The model under review builds one solid part; all positions refer to its coordinate system, in mm. Round coordinates to 2 decimals unless told otherwise and drop trailing zeros. Order: outer loops, then holes, each group sorted by start corner. A loop starts at its lowest first (then second) coordinate and runs counter-clockwise, first axis right, second up.
1) Clearance check with flat-ended pins moving along their axes: P1, Ø1, axis at x = 10, z = 38, coming from the +Y side; P2, Ø5, axis at x = 2.5, z = 35, coming from the -Y side; P3, Ø10, axis at x = -1.5, y = 10.5, coming from the +Z side. State where each tip first meets the part, or that it passes through.
2) Mouldability with a two-part tool opening along Y and no side actions: class faces 1 (the face through (0, 0, 0)), 2 (the face through (-29.97, 1.32, 33.28)), 3 (the face through (0, 0, 7)) as pulls with the +Y half, pulls with the -Y half, needs draft (parallel to the pull), parting line crosses it, or undercut.
3) To check wall thickness, follow L1, parallel to Y at x = 0, z = 61; L2, parallel to Z at x = 23, y = 1; L3, parallel to Y at x = 8.5, z = 64. State the ranges of each line that lie inside material, in increasing order.
4) Consider section A-A (x = 0). Give the boundary of the cut face in (y, z).
5) Consider section C-C (z = 58.5). Give the boundary of the cut face in (x, y).
from build123d import *

# Parameters (mm, degrees)
F0_R     = 30
F0_R_2   = 25
F1_DEPTH = 70
F2_DEPTH = 7
F3_R     = 2.5


# Not quite as in the source:
# - a fillet or chamfer that OpenCascade refuses, or shapes differently, is made with other operations: its cross-section is extruded or revolved along the edge and cut away or added


with BuildPart() as f1:
    # F0 (on Top) → F1 (new body)
    with BuildSketch(Plane.XY):
        Circle(F0_R)
        Circle(F0_R_2, mode=Mode.SUBTRACT)
    extrude(amount=F1_DEPTH)

    # F0 (on Top) → F2 (join)
    with BuildSketch(Plane.XY):
        Circle(F0_R_2)
    extrude(amount=F2_DEPTH)

    # F3
    f3_edges = [f1.edges().sort_by_distance(p)[0] for p in [
        (-30, 0, 70),
    ]]
    fillet(f3_edges, radius=F3_R)

    # F4: fillet of radius 4.8284271247 on 1 edges, made by hand

    # F4_s1 → F4_t2 (revolve, cut)
    with BuildSketch(Plane.XZ):
        with BuildLine():
            ThreePointArc((27.5, 70), (25.6717247547, 68.2268227163), (25, 65.7700903528))
            Line((25, 65.7700903528), (24.9034314575, 65.7700903528))
            Line((24.9034314575, 65.7700903528), (24.9034314575, 70))
            Line((24.9034314575, 70), (25, 70.0965685425))
            ThreePointArc((25, 70.0965685425), (26.25, 70.0965685425), (27.4534314575, 70.0845981929))
            Line((27.4534314575, 70.0845981929), (27.5, 70))
        make_face()
    revolve(axis=Axis((0, 0, 70), (0, 0, 1)), mode=Mode.SUBTRACT)


solid = f1.part
Answer below:
1. P1: stops at y = 28.46
1. P2: stops at y = -30
1. P3: stops at z = 7
2. face 1: needs draft
2. face 2: parting line crosses it
2. face 3: undercut
3. L1: y = -30 to -25, 25 to 30
3. L2: z = 0 to 7
3. L3: y = -28.77 to -23.51, 23.51 to 28.77
4. outline: (-30, 0) - (30, 0) - (30, 67.5) arc R2.5 ccw to (27.5, 70) arc R4.83 ccw to (25, 65.77) - (25, 7) - (-25, 7) - (-25, 65.77) arc R4.83 ccw to (-27.5, 70) arc R2.5 ccw to (-30, 67.5) - close
5. outline: circle Ø60 at (0, 0); hole circle Ø50 at (0, 0)
